```python
from build123d import *
from build123d.topology import SkipClean

# Parameters (mm, degrees)
EXTRUDE_1_DEPTH     = 9
SKETCH_2_R          = 5.6
CUT_EXTRUDE_1_DEPTH = 4.6
SKETCH_3_R          = 2.6
CUT_EXTRUDE_2_DEPTH = 178.798114195
SKETCH_5_W          = 132.43986789
SKETCH_5_H          = 5.139725872
CUT_EXTRUDE_3_DEPTH = 181.463576917
EXTRUDE_START       = -7.270147681
SKETCH_6_R          = 4.358898944
EXTRUDE_2_DEPTH     = 7.270147681
SKETCH_7_R          = 4.358898944
EXTRUDE_3_DEPTH     = 7.270147681
SKETCH_8_R          = 2.5
EXTRUDE_4_DEPTH     = 2
CUT_EXTRUDE_4_REACH = 179.798
SKETCH_9_R          = 1.75


with BuildPart() as part:
    # 草图1 → 凸台-拉伸1 (new body)
    with BuildSketch(Plane.XY):
        with BuildLine():
            Line((97.080968947, -107.358898944), (137.080968947, -107.358898944))
            ThreePointArc((137.080968947, -107.358898944), (141.43986789, -103), (137.080968947, -98.641101056))
            Line((137.080968947, -98.641101056), (100.473705575, -98.641101056))
            Line((100.473705575, -98.641101056), (75.225539013, 1.069962639))
            ThreePointArc((75.225539013, 1.069962639), (73.67732525, 3.439757187), (71, 4.358898944))
            Line((71, 4.358898944), (9, 4.358898944))
            ThreePointArc((9, 4.358898944), (-10, 0), (9, -4.358898944))
            Line((9, -4.358898944), (67.607263372, -4.358898944))
            Line((67.607263372, -4.358898944), (92.855429934, -104.069962639))
            ThreePointArc((92.855429934, -104.069962639), (94.403643697, -106.439757187), (97.080968947, -107.358898944))
        make_face()
    extrude(amount=EXTRUDE_1_DEPTH)

    # 草图2 → 切除-拉伸1 (cut)
    with BuildSketch(Plane(origin=(0, 0, 0), x_dir=(-1, 0, 0), z_dir=(0, 0, -1))):
        Circle(SKETCH_2_R)
    extrude(amount=-CUT_EXTRUDE_1_DEPTH, mode=Mode.SUBTRACT)

    # 草图3 → 切除-拉伸2 (cut, through all)
    with BuildSketch(Plane.XY.offset(9)):
        Circle(SKETCH_3_R)
    extrude(amount=-CUT_EXTRUDE_2_DEPTH, mode=Mode.SUBTRACT)

    # 草图5 → 切除-拉伸3 (cut, through all)
    with BuildSketch(Plane(origin=(0, 4.358898944, 0), x_dir=(1, 0, 0), z_dir=(0, 1, 0))):
        with Locations((75.219933945, -4.299715255)):
            Rectangle(SKETCH_5_W, SKETCH_5_H)
    extrude(amount=-CUT_EXTRUDE_3_DEPTH, mode=Mode.SUBTRACT)

    # 草图6 → 凸台-拉伸2 (add)
    with SkipClean():  # the faces are left unmerged after this step: merging them gives an invalid solid
        with BuildSketch(Plane.XY.offset(9).offset(EXTRUDE_START)):
            with Locations(Location((71, 0, 0), (0, 0, 90))):
                Circle(SKETCH_6_R)
        extrude(amount=EXTRUDE_2_DEPTH)

    # 草图7 → 凸台-拉伸3 (add)
    with SkipClean():  # the faces are left unmerged after this step: merging them gives an invalid solid
        with BuildSketch(Plane.XY.offset(9).offset(EXTRUDE_START)):
            with Locations(Location((97.080968947, -103, 0), (0, 0, 194.209390146))):
                Circle(SKETCH_7_R)
        extrude(amount=EXTRUDE_3_DEPTH)

    # 草图8 → 凸台-拉伸4 (add)
    with SkipClean():  # the faces are left unmerged after this step: merging them gives an invalid solid
        with BuildSketch(Plane.XY.offset(1.729852319)):
            with Locations(Location((137.080968947, -103, 0), (0, 0, 180))):
                Circle(SKETCH_8_R)
        extrude(amount=EXTRUDE_4_DEPTH)

    # 草图9 → 切除-拉伸4 (cut, up to next)
    with BuildSketch(Plane.XY.offset(9), mode=Mode.PRIVATE) as cut_extrude_4_sk1:
        with Locations((137.080968947, -103)):
            Circle(SKETCH_9_R)
    cut_extrude_4_tool1 = extrude(cut_extrude_4_sk1.sketch, amount=-CUT_EXTRUDE_4_REACH, mode=Mode.PRIVATE) & part.part
    add(cut_extrude_4_tool1.solids().sort_by_distance((137.080969, -103, 9))[0], mode=Mode.SUBTRACT)


solid = part.part
```
Here's how the part is built. I have some questions about the finished solid (model axes, mm). A direction names the side the tool comes from. Round coordinates to 2 decimals unless told otherwise and drop trailing zeros. Order: outer loops, then holes, each group sorted by start corner. A loop starts at its lowest first (then second) coordinate and runs counter-clockwise, first axis right, second up. Notation, with made-up numbers: M 15.5,42.5 L 58.5,42.5 A26 cw 58.5,68.5 Z; hole C -8,31.5 d7. An arc over 180 degrees is marked long. One line per question, with ' | ' between items.
1) I need wall thicknesses on line 1 along Z through (x, y) = (109, -102); line 2 along Y through (x, z) = (0, 1.05); line 3 along X through (y, z) = (4, 2.25). Which ranges of each line are inside material? Lowest first, please.
Working result:
line 1: 0 to 1.73, 6.87 to 9 | line 2: -10 to -5.6, 5.6 to 10 | line 3: -9.17 to -3.92, 3.92 to 9, 69.27 to 72.73
2) For pin 1 Ø0.5 at (x, z) = (112.5, 1) entering from +Y; pin 2 Ø1.1 at (x, z) = (31, 7.5) entering from +Y; pin 3 Ø1.1 at (x, z) = (25, 8.5) entering from -Y, each with a flat end and sliding along its axis, tell me the tip position at first contact or that it passes through.
Working result:
pin 1: y = -98.64 | pin 2: y = 4.36 | pin 3: y = -4.36
3) If we mould it in two halves opening along X, with no side actions, what happens to faces 1 (the face through (88.026, -49.484, 7.92)), 2 (the face through (3, -1, 4.6)), 3 (the face through (77, -40, 0))? For each: +X half, -X half, draft (parallel to the pull), parting line (faces both ways), or undercut.
Working result:
face 1: +X half | face 2: undercut | face 3: draft
4) I want a section at B-B, the plane x = 85. Write out the boundary of the cut face in (y, z).
Working result:
outline: M -73.05,0 L -37.53,0 L -37.53,1.73 L -73.05,1.73 Z; M -73.05,6.87 L -37.53,6.87 L -37.53,9 L -73.05,9 Z
5) I want a section at A-A, the plane y = -74. Write out the boundary of the cut face in (x, z).
Working result:
outline: M 85.24,0 L 94.23,0 L 94.23,1.73 L 85.24,1.73 Z; M 85.24,6.87 L 94.23,6.87 L 94.23,9 L 85.24,9 Z
6) For faces 4 (the face through (134.696, -103.751, 2.716)), 5 (the face through (135.69, -104.06, 7.95)), 6 (the face through (5.595, 0.246, 2.268)), 7 (the face through (137, -103, 3.73)), 8 (the face through (9, 0, 4)), which set-ups out of +Z, -Z, +X, -X, +Y, -Y let a thin tool reach every point of the face, with its end or its side?
Working result:
face 4: none | face 5: +Z | face 6: -Z | face 7: +X, +Y, -Y | face 8: +Y, -Y
